Geometry check sheet. Reference: the model listing, model coordinates, mm. A direction names the side the tool comes from. Round coordinates to 2 decimals unless told otherwise and drop trailing zeros. Order: outer loops, then holes, each group sorted by start corner. A loop starts at its lowest first (then second) coordinate and runs counter-clockwise, first axis right, second up.
(1) Cross-section at B-B on z = -6. Enter the section's corners in (x, y).
(2) Gauge pin test, flat ends, axial feed: P1, Ø2, axis at x = -45.5, y = -73.5, coming from the +Z side; P2, Ø6, axis at y = -187.5, z = -37.5, coming from the -X side; P3, Ø2, axis at y = -313, z = -45.5, coming from the +X side; P4, Ø4, axis at x = 17.5, z = -45, coming from the +Y side. Record the tip position at first contact, or that the pin passes through.
(3) Set-up check for faces 1 (the face through (50, -86.617, -30)), 2 (the face through (-63, -239, -2.318)), 3 (the face through (-1, -217, -48.102)), 4 (the face through (70, -239, -2.318)): record each of +Z, -Z, +X, -X, +Y, -Y from which the full face is reachable in a straight line by a thin tool's end or side.
(4) Cross-section at C-C on x = 34.5. Enter the section's corners in (y, z).
(5) Cross-section at A-A on y = -181. Enter the section's corners in (x, z), and give its area (3 significant figures).
(6) Draft check along X on faces 5 (the face through (-54.997, -103.412, -7.525)), 6 (the face through (-50.35, -216.71, -27.34)), 7 (the face through (-47.52, -216.71, -23.04)). Enter one of: pulls with the +X half, pulls with the -X half, needs draft (parallel to the pull), parting line crosses it, or undercut.
(7) Thickness scan on L1, parallel to Z at x = 33.5, y = -315; L2, parallel to Z at x = -58, y = -215.5; L3, parallel to X at y = -131, z = -8. Record the ranges inside material, lowest first.
from build123d import *

# Parameters (mm, degrees)
F0_W     = 143
F0_H     = 53
F1_DEPTH = 365
F3_DEPTH = 143.001
F5_DEPTH = 300.785325
F6_DEPTH = 300.785325


with BuildPart() as f1:
    # F0 (on Front) → F1 (new body)
    with BuildSketch(Plane.XZ):
        with Locations((3.823606, -25.164385)):
            Rectangle(F0_W, F0_H)
    extrude(amount=F1_DEPTH)

    # F2 (on face) → F3 (cut, through all)
    with BuildSketch(Plane(origin=(-67.676394, 0, 0), x_dir=(0, -1, 0), z_dir=(-1, 0, 0))):
        Polygon((0, -51.664385), (64.215675, -51.664385), (64.215675, -37.959635), (86.616777, -37.959635), (86.616777, -21.311939), (114.20504, 1.335615), (0, 1.335615), (0, -16.486794), (0, -25.164385), align=None)
    extrude(amount=-F3_DEPTH, mode=Mode.SUBTRACT)

    # F4 (on face) → F5 (cut, through all)
    with BuildSketch(Plane.XZ.offset(365)):
        Polygon((-57.691015, -2.318196), (-67.676394, -2.318196), (-67.676394, -51.664385), (-43.213006, -51.664385), align=None)
        Polygon((65.37208, -2.318196), (41.786994, -51.664385), (75.323606, -51.664385), (75.323606, -2.318196), align=None)
    extrude(amount=-F5_DEPTH, mode=Mode.SUBTRACT)

    # F4 (on face) → F6 (cut, through all)
    with BuildSketch(Plane.XZ.offset(365)):
        Polygon((62.925503, 1.335615), (-54.888126, 1.335615), (-39.947845, -48.101962), (39.710268, -48.101962), align=None)
    extrude(amount=-F6_DEPTH, mode=Mode.SUBTRACT)


solid = f1.part
Found:
1. outline: (-56.61, -365) - (-52.67, -365) - (-52.67, -105.27) - (-56.61, -105.27) - close; (59.48, -365) - (63.61, -365) - (63.61, -105.27) - (59.48, -105.27) - close
2. P1: stops at z = -37.96
2. P2: stops at x = -48.25
2. P3: stops at x = 45.21
2. P4: passes through
3. face 1: +Z, +X, -X, +Y
3. face 2: -Z, -X, +Y, -Y
3. face 3: +Z, +Y, -Y
3. face 4: -Z, +X, +Y, -Y
4. outline: (-365, -51.66) - (-64.22, -51.66) - (-64.22, -48.1) - (-365, -48.1) - close
5. outline: (-67.68, -2.32) - (-57.69, -2.32) - (-43.21, -51.66) - (41.79, -51.66) - (65.37, -2.32) - (75.32, -2.32) - (75.32, 1.34) - (62.93, 1.34) - (39.71, -48.1) - (-39.95, -48.1) - (-54.89, 1.34) - (-67.68, 1.34) - close
5. area: 775 mm2
6. face 5: needs draft
6. face 6: pulls with the -X half
6. face 7: undercut
7. L1: z = -51.66 to -48.1
7. L2: z = -2.32 to 1.34
7. L3: x = -56.02 to -52.07, 58.54 to 62.66
